from build123d import *

# Parameters (mm, degrees)
SKETCH_1_W      = 65
SKETCH_1_H      = 65
SKETCH_1_R      = 2.15
EXTRUDE_1_DEPTH = 5
SKETCH_3_W      = 11.26
SKETCH_3_H      = 11.26
EXTRUDE_2_DEPTH = 120
SKETCH_4_W      = 65
SKETCH_4_H      = 65
SKETCH_4_R      = 2
EXTRUDE_3_DEPTH = 5
FILLET_1_R      = 10
FILLET_5_R      = 3
EXTRUDE_4_DEPTH = 10
FILLET_6_R      = 10
FILLET_8_R      = 5
FILLET_9_R      = 5
FILLET_10_R     = 5
FILLET_11_R     = 5
FILLET_12_R     = 5


# Some blends are built 0.0001 mm under size
with BuildPart() as part:
    # 草图1 → 凸台-拉伸1 (new body)
    with BuildSketch(Plane.XY):
        Rectangle(SKETCH_1_W, SKETCH_1_H)
        with Locations((-26.87, 26.87)):
            Circle(SKETCH_1_R, mode=Mode.SUBTRACT)
        with Locations(Location((26.87, 26.87, 0), (0, 0, 180))):
            Circle(SKETCH_1_R, mode=Mode.SUBTRACT)
        with Locations((26.87, -26.87)):
            Circle(SKETCH_1_R, mode=Mode.SUBTRACT)
        with Locations(Location((-26.87, -26.87, 0), (0, 0, 180))):
            Circle(SKETCH_1_R, mode=Mode.SUBTRACT)
    extrude(amount=EXTRUDE_1_DEPTH)

    # 草图3 → 凸台-拉伸2 (add)
    with BuildSketch(Plane.XY.offset(5)):
        with Locations((-26.87, 26.87)):
            Rectangle(SKETCH_3_W, SKETCH_3_H)
        with Locations((26.87, 26.87)):
            Rectangle(SKETCH_3_W, SKETCH_3_H)
        with Locations((26.87, -26.87)):
            Rectangle(SKETCH_3_W, SKETCH_3_H)
        with Locations((-26.87, -26.87)):
            Rectangle(SKETCH_3_W, SKETCH_3_H)
    extrude(amount=EXTRUDE_2_DEPTH)

    # 草图4 → 凸台-拉伸3 (add)
    with BuildSketch(Plane.XY.offset(125)):
        Rectangle(SKETCH_4_W, SKETCH_4_H)
        with Locations((0, 7)):
            Circle(SKETCH_4_R, mode=Mode.SUBTRACT)
        with Locations((7, 0)):
            Circle(SKETCH_4_R, mode=Mode.SUBTRACT)
        with Locations((-7, 0)):
            Circle(SKETCH_4_R, mode=Mode.SUBTRACT)
    extrude(amount=EXTRUDE_3_DEPTH)

    # 圆角1
    fillet_1_edges = [part.edges().sort_by_distance(p)[0] for p in [
        (-26.87, 21.24, 5),
        (-21.24, 26.87, 5),
        (21.24, 26.87, 5),
        (26.87, 21.24, 5),
        (21.24, -26.87, 5),
        (26.87, -21.24, 5),
        (-21.24, -26.87, 5),
        (-26.87, -21.24, 5),
    ]]
    fillet(fillet_1_edges, radius=FILLET_1_R)

    # 圆角5
    fillet_5_edges = [part.edges().sort_by_distance(p)[0] for p in [
        (-32.5, 0, 130),
        (0, -32.5, 130),
        (32.5, 0, 130),
        (0, 32.5, 130),
    ]]
    fillet(fillet_5_edges, radius=FILLET_5_R)

    # 草图6 → 凸台-拉伸4 (add)
    with BuildSketch(Plane(origin=(0, 0, 125), x_dir=(-1, 0, 0), z_dir=(0, 0, -1))):
        Polygon((32.5, 21.24), (21.24, 21.24), (21.24, 32.5), (-21.24, 32.5), (-21.24, 21.24), (-32.5, 21.24), (-32.5, -21.24), (-21.24, -21.24), (-21.24, -32.5), (21.24, -32.5), (21.24, -21.24), (32.5, -21.24), align=None)
    extrude(amount=EXTRUDE_4_DEPTH)

    # 圆角6
    fillet_6_edges = [part.edges().sort_by_distance(p)[0] for p in [
        (-26.87, 21.24, 115),
        (-21.24, 26.87, 115),
        (21.24, 26.87, 115),
        (26.87, 21.24, 115),
        (26.87, -21.24, 115),
        (21.24, -26.87, 115),
        (-21.24, -26.87, 115),
        (-26.87, -21.24, 115),
    ]]
    fillet(fillet_6_edges, radius=FILLET_6_R)

    # 圆角8
    fillet_8_edges = [part.edges().sort_by_distance(p)[0] for p in [
        (0, 32.5, 5),
        (-18.311067812, 32.5, 7.928932188),
        (18.311067812, 32.5, 7.928932188),
        (0, 32.5, 115),
        (-21.24, 32.5, 60),
        (21.24, 32.5, 60),
        (-18.311067812, 32.5, 112.071067812),
        (18.311067812, 32.5, 112.071067812),
    ]]
    fillet(fillet_8_edges, radius=FILLET_8_R - 0.0001)  # a hair under: the kernel refuses the full size

    # 圆角9
    fillet_9_edges = [part.edges().sort_by_distance(p)[0] for p in [
        (32.5, 0, 5),
        (32.5, 18.311067812, 7.928932188),
        (32.5, -18.311067812, 7.928932188),
        (32.5, 0, 115),
        (32.5, -21.24, 60),
        (32.5, 21.24, 60),
        (32.5, -18.311067812, 112.071067812),
        (32.5, 18.311067812, 112.071067812),
    ]]
    fillet(fillet_9_edges, radius=FILLET_9_R - 0.0001)  # a hair under: the kernel refuses the full size

    # 圆角10
    fillet_10_edges = [part.edges().sort_by_distance(p)[0] for p in [
        (0, -32.5, 5),
        (-18.311067812, -32.5, 7.928932188),
        (18.311067812, -32.5, 7.928932188),
        (0, -32.5, 115),
        (-21.24, -32.5, 60),
        (21.24, -32.5, 60),
        (-18.311067812, -32.5, 112.071067812),
        (18.311067812, -32.5, 112.071067812),
    ]]
    fillet(fillet_10_edges, radius=FILLET_10_R - 0.0001)  # a hair under: the kernel refuses the full size

    # 圆角11
    fillet_11_edges = [part.edges().sort_by_distance(p)[0] for p in [
        (-32.5, 0, 5),
        (-32.5, -18.311067812, 7.928932188),
        (-32.5, 18.311067812, 7.928932188),
        (-32.5, 0, 115),
        (-32.5, -21.24, 60),
        (-32.5, 21.24, 60),
        (-32.5, -18.311067812, 112.071067812),
        (-32.5, 18.311067812, 112.071067812),
    ]]
    fillet(fillet_11_edges, radius=FILLET_11_R - 0.0001)  # a hair under: the kernel refuses the full size

    # 圆角12
    # the kernel refuses this fillet: 5 mm, written as the material it takes off along each edge
    with BuildSketch(Plane(origin=(-27.5, -27.5, 130), x_dir=(-1, 0, 0), z_dir=(0, 1, 0))) as fillet_12_piece_1:
        with BuildLine():
            CenterArc((2, -3), 3, 0, 90)
            Line((5, -3), (5, 0))
            Line((5, 0), (2, 0))
        make_face()
    revolve(axis=Axis((-27.5, -27.5, 130), (0, 0, 1)), revolution_arc=90, mode=Mode.SUBTRACT)
    with BuildSketch(Plane(origin=(-27.5, 27.5, 130), x_dir=(0, 1, 0), z_dir=(1, 0, 0))) as fillet_12_piece_2:
        with BuildLine():
            CenterArc((2, -3), 3, 0, 90)
            Line((5, -3), (5, 0))
            Line((5, 0), (2, 0))
        make_face()
    revolve(axis=Axis((-27.5, 27.5, 130), (0, 0, 1)), revolution_arc=90, mode=Mode.SUBTRACT)
    with BuildSketch(Plane(origin=(27.5, -27.5, 130), x_dir=(0, -1, 0), z_dir=(-1, 0, 0))) as fillet_12_piece_3:
        with BuildLine():
            CenterArc((2, -3), 3, 0, 90)
            Line((5, -3), (5, 0))
            Line((5, 0), (2, 0))
        make_face()
    revolve(axis=Axis((27.5, -27.5, 130), (0, 0, 1)), revolution_arc=90, mode=Mode.SUBTRACT)
    with BuildSketch(Plane(origin=(27.5, 27.5, 130), x_dir=(1, 0, 0), z_dir=(0, -1, 0))) as fillet_12_piece_4:
        with BuildLine():
            CenterArc((2, -3), 3, 0, 90)
            Line((5, -3), (5, 0))
            Line((5, 0), (2, 0))
        make_face()
    revolve(axis=Axis((27.5, 27.5, 130), (0, 0, 1)), revolution_arc=90, mode=Mode.SUBTRACT)
    with BuildSketch(Plane(origin=(32.5, 32.5, 130), x_dir=(-1, 0, 0), z_dir=(0, 0, -1)), Plane(origin=(-32.5, -32.5, -12.5), x_dir=(0, 1, 0), z_dir=(0, 0, 1))) as fillet_12_piece_5:
        with BuildLine():
            CenterArc((FILLET_12_R, -FILLET_12_R), FILLET_12_R, 90, 90)
            Line((0, -FILLET_12_R), (0, 0))
            Line((0, 0), (FILLET_12_R, 0))
        make_face()
    extrude(amount=142.5, mode=Mode.SUBTRACT)
    with BuildSketch(Plane(origin=(32.5, -32.5, 130), x_dir=(-1, 0, 0), z_dir=(0, 0, -1)), Plane(origin=(-32.5, 32.5, -12.5), x_dir=(0, -1, 0), z_dir=(0, 0, 1))) as fillet_12_piece_6:
        with BuildLine():
            CenterArc((FILLET_12_R, FILLET_12_R), FILLET_12_R, 180, 90)
            Line((0, FILLET_12_R), (0, 0))
            Line((0, 0), (FILLET_12_R, 0))
        make_face()
    extrude(amount=142.5, mode=Mode.SUBTRACT)


solid = part.part
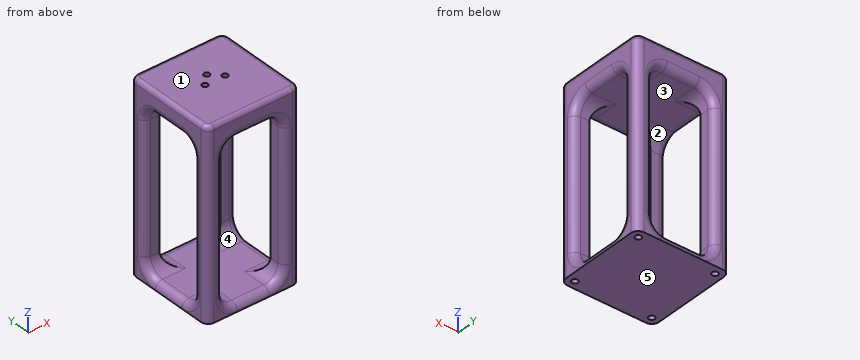
Can you work these out from the model? Positions are in its coordinate system, mm. Face numbers are marked on the shaded views. A direction names the side the tool comes from. Coordinates: 2 decimals unless noted, no trailing zeros. Loops run counter-clockwise (first coordinate to the right, second up) from the corner with the lowest first, then second, coordinate; pieces in that order, holes last. Notation, with made-up numbers: M -6.75,3.5 L -1.75,3.5 A38 ccw -1.75,41.5 Z; hole C -8,26 d10. An arc over 180 degrees is marked long. Return JSON: item names as keys, results as strings. Group by question number.
Item 1: Imagine slicing it at B-B (z = 100.5). Please give me the cut outline in (x, y), and give its area (3 significant figures).
Item 2: If I drill on L1, parallel to Y at x = -26.87, z = 1.8; L2, parallel to Z at x = 2, y = -27; L3, parallel to Y at x = 26, z = 3, over which ranges is the centre line in solid material (lowest first)? Write a range as from..to.
Item 3: On a 3-axis mill with a long thin cutter (end or side, diameter ignored), from which of +Z, -Z, +X, -X, +Y, -Y can I reach the whole of each face in a straight line? I mean the marked faces 3, 4 and 5. Say none if no direction works.
Item 4: I'm going to push flat-ended pins straight in: pin 1 Ø1.9 at (x, z) = (24, 46.5) entering from +Y; pin 2 Ø2 at (x, y) = (-6.5, -0.5) entering from +Z; pin 3 Ø1.9 at (x, z) = (-23.5, 71.5) entering from +Y. Where does each tip first touch, or does it pass through?
Item 5: Thinking about a two-plate mould opening in Y: for the marked faces 1 and 2, which applies, released by +Y, released by -Y, zero draft, split by the parting line, or undercut?
Verdict:
{
 "1": {"outline": "M -32.5,-27.5 A5 ccw -27.5,-32.5 L -26.24,-32.5 A5 ccw -21.24,-27.5 L -21.24,-21.24 L -27.5,-21.24 A5 ccw -32.5,-26.24 Z; M -32.5,26.24 A5 ccw -27.5,21.24 L -21.24,21.24 L -21.24,27.5 A5 ccw -26.24,32.5 L -27.5,32.5 A5 ccw -32.5,27.5 Z; M 21.24,-27.5 A5 ccw 26.24,-32.5 L 27.5,-32.5 A5 ccw 32.5,-27.5 L 32.5,-26.24 A5 ccw 27.5,-21.24 L 21.24,-21.24 Z; M 21.24,21.24 L 27.5,21.24 A5 ccw 32.5,26.24 L 32.5,27.5 A5 ccw 27.5,32.5 L 26.24,32.5 A5 ccw 21.24,27.5 Z", "area": "443 mm^2"},
 "2": {"L1": "y = -32.5..-29.02, -24.72..24.72, 29.02..32.5", "L2": "z = 0..5, 115..130", "L3": "y = -32.5..-28.84, -24.9..24.9, 28.84..32.5"},
 "3": {"face 3": "none", "face 4": "+X, -X", "face 5": "-Z, +X, -X, +Y, -Y"},
 "4": {"pin 1": "stops at y = 32.33", "pin 2": "stops at z = 125", "pin 3": "stops at y = 32.17"},
 "5": {"face 1": "zero draft", "face 2": "undercut"}
}
